```python
from build123d import *

# Parameters (mm, degrees)
SKETCH1_R           = 8
SKETCH1_R_2         = 1.65
SKETCH1_R_3         = 10.25
BOSS_EXTRUDE1_DEPTH = 4
SKETCH4_R           = 8
SKETCH4_R_2         = 4.15
BOSS_EXTRUDE3_DEPTH = 2
SKETCH5_R           = 10
SKETCH5_R_2         = 4.1
BOSS_EXTRUDE4_DEPTH = 2
FILLET6_R           = 2


with BuildPart() as part:
    # Sketch1 → Boss-Extrude1 (new body)
    with BuildSketch(Plane(origin=(0, 0, 0), x_dir=(1, 0, 0), z_dir=(0, 1, 0))):
        with BuildLine():
            Line((-3.333333333, 19.720265944), (-50, 11.832159566))
            ThreePointArc((-50, 11.832159566), (-60, 0), (-50, -11.832159566))
            Line((-50, -11.832159566), (-3.333333333, -19.720265944))
            ThreePointArc((-3.333333333, -19.720265944), (20, 0), (-3.333333333, 19.720265944))
        make_face()
        with Locations(Location((-48, 0, 0), (0, 0, 270))):
            Circle(SKETCH1_R, mode=Mode.SUBTRACT)
        with Locations(Location((-7.5, -12.990381057, 0), (0, 0, 270))):
            Circle(SKETCH1_R_2, mode=Mode.SUBTRACT)
        with Locations(Location((7.5, -12.990381057, 0), (0, 0, 270))):
            Circle(SKETCH1_R_2, mode=Mode.SUBTRACT)
        with Locations(Location((15, 0, 0), (0, 0, 270))):
            Circle(SKETCH1_R_2, mode=Mode.SUBTRACT)
        with BuildLine():
            ThreePointArc((-13.35, 0), (-15, -1.65), (-16.65, 0))
            ThreePointArc((-16.65, 0), (-15, 1.65), (-13.35, 0))
        make_face(mode=Mode.SUBTRACT)
        with Locations(Location((0, 0, 0), (0, 0, 270))):
            Circle(SKETCH1_R_3, mode=Mode.SUBTRACT)
        with Locations(Location((-7.5, 12.990381057, 0), (0, 0, 270))):
            Circle(SKETCH1_R_2, mode=Mode.SUBTRACT)
        with Locations(Location((7.5, 12.990381057, 0), (0, 0, 270))):
            Circle(SKETCH1_R_2, mode=Mode.SUBTRACT)
    extrude(amount=BOSS_EXTRUDE1_DEPTH)



with BuildPart() as body_2:
    # Sketch4 → Boss-Extrude3 (new body)
    with BuildSketch(Plane.XZ):
        with Locations(Location((-48, 0, 0), (0, 0, 90))):
            Circle(SKETCH4_R)
        with Locations(Location((-48, 0, 0), (0, 0, 270))):
            Circle(SKETCH4_R_2, mode=Mode.SUBTRACT)
    extrude(amount=BOSS_EXTRUDE3_DEPTH)


with BuildPart() as part_1:
    add(part.part)

    add(body_2.part)  # Boss-Extrude4 merges body 2
    # Sketch5 → Boss-Extrude4 (add)
    with BuildSketch(Plane.XZ):
        with Locations(Location((-48, 0, 0), (0, 0, 90))):
            Circle(SKETCH5_R)
        with Locations(Location((-48, 0, 0), (0, 0, 270))):
            Circle(SKETCH5_R_2, mode=Mode.SUBTRACT)
    extrude(amount=BOSS_EXTRUDE4_DEPTH)

    # Fillet6
    fillet6_edges = [part_1.edges().sort_by_distance(p)[0] for p in [
        (-48, 0, -10),
    ]]
    fillet(fillet6_edges, radius=FILLET6_R - 0.0001)  # a hair under: the kernel refuses the full size


solid = part_1.part
```
CAD build for the part. Positions are in the model's coordinates, mm. A direction names the side the tool comes from. Give positions to 0.01 mm unless a question says otherwise; leave off trailing zeros. Loops run counter-clockwise (first coordinate to the right, second up) from the corner with the lowest first, then second, coordinate; pieces in that order, holes last. Notation, with made-up numbers: (-39.75, -21.5) - (-20.75, -21.5) arc R18 cw to (-20.75, -5.5) - close; hole circle Ø5 at (17, 69). An arc over 180 degrees is marked (long way). Put each result on its own line as item: value.
Q1. Mould opens along X. For faces 3 (the face through (-26.99, 1.97, 15.72)), 4 (the face through (-12, 0, 0)), 5 (the face through (-8.504, 1.972, -14.3)) say: pulls with the +X half, pulls with the -X half, needs draft (parallel to the pull), parting line crosses it, or undercut.
Filled in:
face 3: pulls with the -X half
face 4: needs draft
face 5: undercut
Q2. Slice it at B-B (z = 0). Give the number of separate pieces and of enclosed holes in the cut face, plus the area to 3 significant figures.
Filled in:
separate pieces: 5
enclosed holes: 0
area: 173 mm²
Q3. Slice it at D-D (z = 13). Give the cut face in (x, y), plus the area to 3 significant figures.
Filled in:
outline: (-43.09, 0) - (-9.15, 0) - (-9.15, 4) - (-43.09, 4) - close; (-5.85, 0) - (5.85, 0) - (5.85, 4) - (-5.85, 4) - close; (9.15, 0) - (15.2, 0) - (15.2, 4) - (9.15, 4) - close
area: 207 mm²
Q4. Probe line 1 along Z through (x, y) = (-8, 2.05); line 2 along Y through (x, z) = (15, -10); line 3 along Z through (x, y) = (-2, 3.4). List the from-to ranges inside material, lowest first.
Filled in:
line 1: z = -18.93 to -14.56, -11.42 to -6.41, 6.41 to 11.42, 14.56 to 18.93
line 2: y = 0 to 4
line 3: z = -19.9 to -10.05, 10.05 to 19.9
Q5. Flat gauge pins, fed straight in: pin 1 (5 mm diameter, centred on x = -44.5, z = 2, fed in from +Y); pin 2 (5.5 mm diameter, centred on x = -15, z = 0, fed in from -Y); pin 3 (3 mm diameter, centred on y = -0.5, z = -14.5, fed in from +X). Where does each tip first touch, or does it go through?
Filled in:
pin 1: stops at y = 0
pin 2: stops at y = 0
pin 3: stops at x = 15.12
Q6. Slice it at A-A (x = 0). Give the cut face in (y, z).
Filled in:
outline: (0, -20) - (4, -20) - (4, -10.25) - (0, -10.25) - close; (0, 10.25) - (4, 10.25) - (4, 20) - (0, 20) - close
Q7. Tool access for faces 1 (the face through (16.39, 1.97, 0.89)), 2 (the face through (-52, 0, -2)): list every direction of +Z, -Z, +X, -X, +Y, -Y with a clear straight run to the whole face (end or side of a thin tool).
Filled in:
face 1: +Y, -Y
face 2: +Y
